Could you check a few things on this model? Use its own coordinates, in mm. A direction names the side the tool comes from. Coordinates: 2 decimals unless noted, no trailing zeros. Loops run counter-clockwise (first coordinate to the right, second up) from the corner with the lowest first, then second, coordinate; pieces in that order, holes last. Notation, with made-up numbers: M 22.25,23 L 73.25,23 A13 cw 73.25,48 Z; hole C 18.25,54 d6. An arc over 180 degrees is marked long. Write each question's results on one line, items separated by ' | '.
```python
from build123d import *

# Parameters (mm, degrees)
IZIM2_R                     = 80
Y_KSEKLIK_EKSTR_ZYON1_DEPTH = 120
Y_KSEKLIK_EKSTR_ZYON3_START = 10
Y_KSEKLIK_EKSTR_ZYON3_DEPTH = 100
IZIM5_R                     = 5
Y_KSEKLIK_EKSTR_ZYON4_DEPTH = 5
IZIM8_R                     = 7.5
Y_KSEKLIK_EKSTR_ZYON6_DEPTH = 60
Y_KSEKLIK_EKSTR_ZYON7_START = 24
IZIM9_R                     = 10
Y_KSEKLIK_EKSTR_ZYON7_DEPTH = 2
Y_KSEKLIK_EKSTR_ZYON8_START = 12
IZIM10_R                    = 10
Y_KSEKLIK_EKSTR_ZYON8_DEPTH = 2


with BuildPart() as part:
    # Çizim2 → Yükseklik-Ekstrüzyon1 (new body)
    with BuildSketch(Plane.XY):
        Circle(IZIM2_R)
    extrude(amount=Y_KSEKLIK_EKSTR_ZYON1_DEPTH)

    # Çizim3 → Yükseklik-Ekstrüzyon3 (add)
    with BuildSketch(Plane.XY.offset(Y_KSEKLIK_EKSTR_ZYON3_START)):
        with BuildLine():
            ThreePointArc((80, 0), (56.568542608, -56.568542382), (3.2e-07, -80))
            Line((3.2e-07, -80), (80, -80))
            Line((80, -80), (80, 0))
        make_face()
        with BuildLine():
            ThreePointArc((3.2e-07, -80), (-56.568542382, -56.568542608), (-80, 0))
            Line((-80, 0), (-80, -80))
            Line((-80, -80), (3.2e-07, -80))
        make_face()
    extrude(amount=Y_KSEKLIK_EKSTR_ZYON3_DEPTH)

    # Çizim5 → Yükseklik-Ekstrüzyon4 (add)
    with BuildSketch(Plane.XZ.offset(80)):
        with Locations(Location((30, 90, 0), (0, 0, 90))):
            Circle(IZIM5_R)
        with Locations(Location((30, 30, 0), (0, 0, 90))):
            Circle(IZIM5_R)
        with Locations(Location((-30, 90, 0), (0, 0, 90))):
            Circle(IZIM5_R)
        with Locations(Location((-30, 30, 0), (0, 0, 90))):
            Circle(IZIM5_R)
    extrude(amount=Y_KSEKLIK_EKSTR_ZYON4_DEPTH)

    # Çizim8 → Yükseklik-Ekstrüzyon6 (add)
    with BuildSketch(Plane.XY.offset(120)):
        Circle(IZIM8_R)
    extrude(amount=Y_KSEKLIK_EKSTR_ZYON6_DEPTH)

    # Çizim9 → Yükseklik-Ekstrüzyon7 (add)
    with BuildSketch(Plane.XY.offset(120).offset(Y_KSEKLIK_EKSTR_ZYON7_START)):
        Circle(IZIM9_R)
    extrude(amount=-Y_KSEKLIK_EKSTR_ZYON7_DEPTH)

    # Çizim10 → Yükseklik-Ekstrüzyon8 (add)
    with BuildSketch(Plane.XY.offset(144).offset(Y_KSEKLIK_EKSTR_ZYON8_START)):
        Circle(IZIM10_R)
    extrude(amount=-Y_KSEKLIK_EKSTR_ZYON8_DEPTH)


solid = part.part
```
(1) Which directions (+Z, -Z, +X, -X, +Y, -Y) give clear straight access to the entire face, cutting with the end or side of a thin tool? Please do faces 1 (the cylindrical face through (-28.085, -82.465, 94.619)), 2 (the flat face through (64, -64, 10)), 3 (the flat face through (-64, -61, 110)).
Reported:
face 1: -Y | face 2: -Z, +X, -Y | face 3: +Z, -X, -Y
(2) Imagine slicing it at C-C, the plane y = -15. List the corners of the cut face in (x, z) for me.
Reported:
outline: M -80,10 L -78.58,10 L -78.58,0 L 78.58,0 L 78.58,10 L 80,10 L 80,110 L 78.58,110 L 78.58,120 L -78.58,120 L -78.58,110 L -80,110 Z
(3) If we mould it in two halves opening along X, with no side actions, what happens to faces 4 (the cylindrical face through (31.915, -82.465, 94.619)), 5 (the cylindrical face through (-7.493, 0.33, 167.832)), 6 (the flat face through (30, -85, 30))? For each: released by +X, released by -X, zero draft, split by the parting line, or undercut.
Reported:
face 4: undercut | face 5: split by the parting line | face 6: zero draft
(4) Imagine slicing it at B-B, the plane x = -30. List the corners of the cut face in (y, z) for me, and give its area (3 significant figures).
Reported:
outline: M -85,25 L -80,25 L -80,10 L -74.16,10 L -74.16,0 L 74.16,0 L 74.16,120 L -74.16,120 L -74.16,110 L -80,110 L -80,95 L -85,95 L -85,85 L -80,85 L -80,35 L -85,35 Z | area: 18,500 mm2
(5) Imagine slicing it at D-D, the plane z = 130. List the corners of the cut face in (x, y) for me.
Reported:
outline: C 0,0 d15
(6) Imagine slicing it at A-A, the plane z = 90. List the corners of the cut face in (x, y) for me, and give its area (3 significant figures).
Reported:
outline: M -80,-80 L -35,-80 L -35,-85 L -25,-85 L -25,-80 L 25,-80 L 25,-85 L 35,-85 L 35,-80 L 80,-80 L 80,0 A80 ccw -80,0 Z | area: 23,000 mm2
(7) Will these pins go through, and if not, where does the flat tip stop? P1, Ø10, axis at x = 32, z = 54.5, coming from the +Y side; P2, Ø10, axis at y = 28, z = 82.5, coming from the +X side; P3, Ø4, axis at x = -42, z = 90, coming from the -Y side.
Reported:
P1: stops at y = 75.31 | P2: stops at x = 76.62 | P3: stops at y = -80
(8) Please list where these lines run through material, in increasing order: probe 1 along Z at (x, y) = (-72.5, -17); probe 2 along Z at (x, y) = (65, -66.5); probe 3 along Y at (x, z) = (0, 21.5). Write a range as from..to.
Reported:
probe 1: z = 0..120 | probe 2: z = 10..110 | probe 3: y = -80..80
